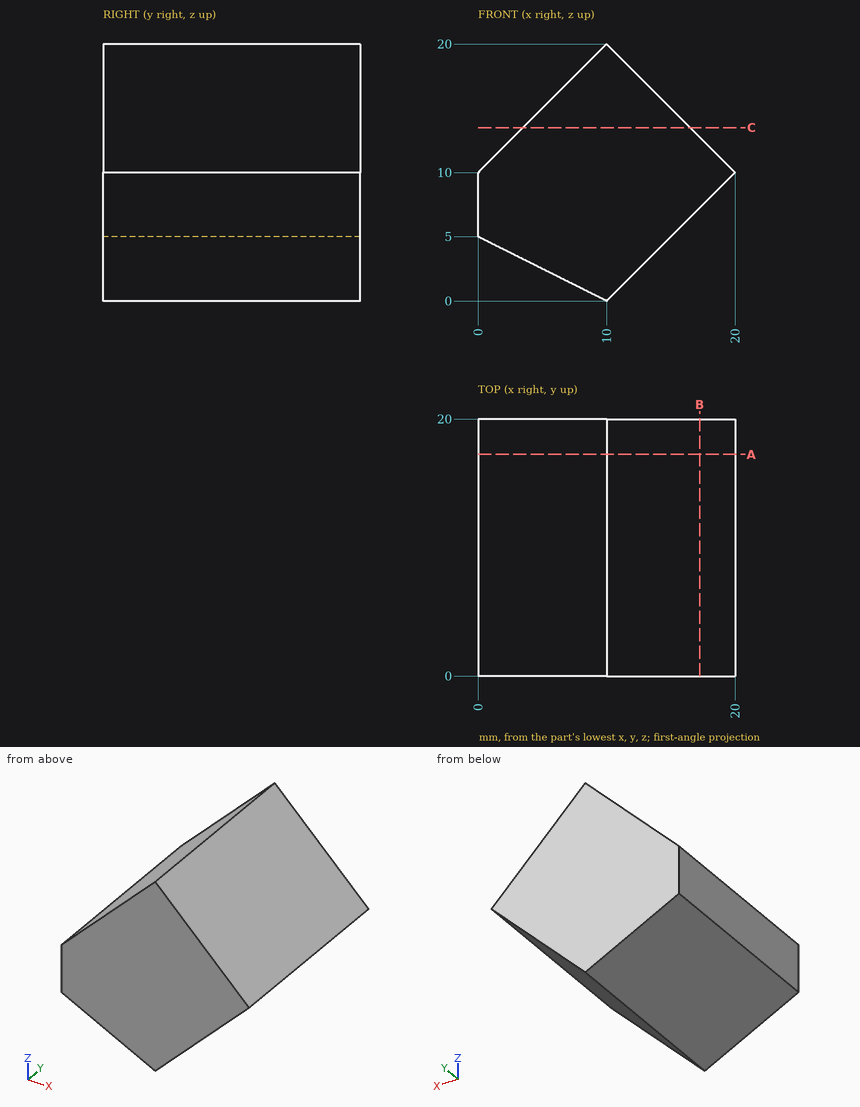
Can you work these out from the drawing? Everything is in mm from the part's minimum corner. Coordinates: 2 decimals unless noted, no trailing zeros. Write each loop counter-clockwise with the first axis right and the second up, starting at its lowest first coordinate (ties: lowest second). Pieces come first, ordered by that corner, then holes. Notation, with made-up numbers: (37, 27.5) - (95, 27.5) arc R11 cw to (95, 45.5) - close; hole circle Ø3 at (-1, 7). An arc over 180 degrees is marked (long way). Use a Markdown table: item, result.
Q1. Imagine slicing it at C-C (z = 13.5). List the corners of the cut face in (x, y) for me, and give its area (3 significant figures).
Geometry check:
| item | result |
|---|---|
| outline | (3.5, 0) - (16.5, 0) - (16.5, 20) - (3.5, 20) - close |
| area | 260 mm2 |
Q2. Imagine slicing it at A-A (y = 17.25). List the corners of the cut face in (x, z) for me, and give its area (3 significant figures).
Geometry check:
| item | result |
|---|---|
| outline | (0, 5) - (10, 0) - (20, 10) - (10, 20) - (0, 10) - close |
| area | 225 mm2 |
Q3. I'm going to push flat-ended pins straight in: pin 1 Ø5 at (y, z) = (15, 6) entering from +X; pin 2 Ø8 at (y, z) = (16.5, 3.5) entering from +X; pin 3 Ø4 at (x, y) = (13.5, 17.5) entering from +Z. Where does each tip first touch, or does it pass through?
Geometry check:
| item | result |
|---|---|
| pin 1 | stops at x = 18.5 |
| pin 2 | stops at x = 17.5 |
| pin 3 | stops at z = 18.5 |
Q4. Please list where these lines run through material, in increasing order: L1, parallel to Z at x = 2.25, y = 19 (3 decimals); L2, parallel to Z at x = 2.5, y = 18.5; L3, parallel to X at y = 2.25, z = 15.5.
Geometry check:
| item | result |
|---|---|
| L1 | z = 3.875 to 12.25 |
| L2 | z = 3.75 to 12.5 |
| L3 | x = 5.5 to 14.5 |
Q5. Imagine slicing it at B-B (x = 17.25). List the corners of the cut face in (y, z) for me.
Geometry check:
| item | result |
|---|---|
| outline | (0, 7.25) - (20, 7.25) - (20, 12.75) - (0, 12.75) - close |
